Can you work these out from the model? Positions are in its coordinate system, mm. Face numbers are marked on the shaded views. A direction names the side the tool comes from. Give positions to 0.01 mm unless a question says otherwise; leave off trailing zeros. Order: outer loops, then holes, each group sorted by start corner. A loop starts at its lowest first (then second) coordinate and runs counter-clockwise, first axis right, second up. Notation, with made-up numbers: (53, -39.5) - (103, -39.5) arc R26 ccw to (103, -0.5) - close; hole circle Ø11 at (63.25, -9.5). An arc over 180 degrees is marked (long way). Use one line per item in the form item = value. Start each with the question number.
1) Please list where these lines run through material, in increasing order: probe 1 along Y at (x, z) = (16, 43.5); probe 2 along Z at (x, y) = (13, -9.5); probe 3 along Y at (x, z) = (-4, 27.5).
2) Suppose I cut it at B-B, the plane y = 28.5. Write out the boundary of the cut face in (x, z), and give its area (3 significant figures).
3) Suppose I cut it at D-D, the plane x = 10.5. Write out the boundary of the cut face in (y, z), and give its area (3 significant figures).
4) We'd pull the mould along X, two halves only. Please class the marked faces 1, 2 and 3: released by +X, released by -X, zero draft, split by the parting line, or undercut.
5) Suppose I cut it at C-C, the plane z = 11. Write out the boundary of the cut face in (x, y).
6) Which directions (+Z, -Z, +X, -X, +Y, -Y) give clear straight access to the entire face, cutting with the end or side of a thin tool? Please do the marked faces 4, 5 and 6.
7) Suppose I cut it at A-A, the plane z = 35. Write out the boundary of the cut face in (x, y), and give its area (3 significant figures).
8) For pin 1 (6.5 mm diameter, centred on x = -6.5, z = 39, fed in from -Y); pin 2 (2 mm diameter, centred on x = 6.5, z = 38, fed in from +Y); pin 3 (13.5 mm diameter, centred on x = -1, y = 31, fed in from +Z), each with a flat end and sliding along its axis, tell me the tip position at first contact or that it passes through.
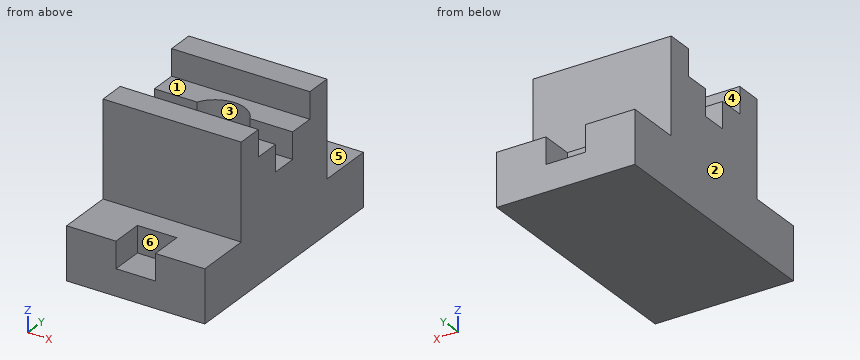
```python
from build123d import *

# Parameters (mm, degrees)
F1_DEPTH = 21
F2_R     = 9
F3_DEPTH = 8
F4_W     = 12
F4_H     = 10
F5_DEPTH = 8


# Not quite as in the source:
# - a pattern or mirror of a feature is missing from the dataset's text; its kind, count and spacing are read off the source's solid


with BuildPart() as f1:
    # F0 (on Right) → F1 (new body, symmetric)
    with BuildSketch(Plane.YZ):
        Polygon((-37, 0), (0, 0), (37, 0), (37, 16), (20, 16), (20, 45), (12, 45), (12, 37), (4, 37), (4, 29), (0, 29), (-4, 29), (-4, 37), (-12, 37), (-12, 45), (-20, 45), (-20, 16), (-37, 16), align=None)
    extrude(amount=F1_DEPTH, both=True)

    # F2 (on face) → F3 (cut, through all)
    with BuildSketch(Plane.XY.offset(37)):
        Circle(F2_R)
    extrude(amount=-F3_DEPTH, mode=Mode.SUBTRACT)

    # F4 (on face) → F5 (cut)
    with BuildSketch(Plane.XY.offset(16)):
        with Locations((0, -32)):
            Rectangle(F4_W, F4_H)
    f5 = extrude(amount=-F5_DEPTH, mode=Mode.SUBTRACT)

    # F5_copies: F5 across plane
    add(f5.mirror(Plane.ZX), mode=Mode.SUBTRACT)


solid = f1.part
```
Result sheet:
q1.probe_1 = -20 to -12, 12 to 20
q1.probe_2 = 0 to 37
q1.probe_3 = -20 to 20
q2.outline = (-21, 0) - (21, 0) - (21, 16) - (6, 16) - (6, 8) - (-6, 8) - (-6, 16) - (-21, 16) - close
q2.area = 576 mm²
q3.outline = (-37, 0) - (37, 0) - (37, 16) - (20, 16) - (20, 45) - (12, 45) - (12, 37) - (4, 37) - (4, 29) - (-4, 29) - (-4, 37) - (-12, 37) - (-12, 45) - (-20, 45) - (-20, 16) - (-37, 16) - close
q3.area = 2,090 mm²
q4.face_1 = zero draft
q4.face_2 = released by -X
q4.face_3 = undercut
q5.outline = (-21, -37) - (-6, -37) - (-6, -27) - (6, -27) - (6, -37) - (21, -37) - (21, 37) - (6, 37) - (6, 27) - (-6, 27) - (-6, 37) - (-21, 37) - close
q6.face_4 = +Z, +X, -X
q6.face_5 = +Z, +X, -X, +Y
q6.face_6 = +Z, -Y
q7.outline = (-21, -20) - (21, -20) - (21, -4) - (8.06, -4) arc R9 cw to (-8.06, -4) - (-21, -4) - close; (-21, 4) - (-8.06, 4) arc R9 cw to (8.06, 4) - (21, 4) - (21, 20) - (-21, 20) - close
q7.area = 1,230 mm²
q8.pin_1 = -20
q8.pin_2 = 20
q8.pin_3 = 16
